```python
from build123d import *

# Parameters (mm, degrees)
SKETCH1_W   = 45.5
SKETCH1_H   = 37
BASIS_DEPTH = 4


with BuildPart() as part:
    # Sketch1 → Basis (new body)
    with BuildSketch(Plane.XY):
        with Locations((22.75, 18.5)):
            Rectangle(SKETCH1_W, SKETCH1_H)
        Polygon((14.5, 39.5), (12.5, 37), (16.5, 37), align=None)
        Polygon((31, 39.5), (29, 37), (33, 37), align=None)
        Polygon((16.5, 0), (12.5, 0), (14.5, -2.5), align=None)
        Polygon((33, 0), (29, 0), (31, -2.5), align=None)
    extrude(amount=BASIS_DEPTH)


solid = part.part
```
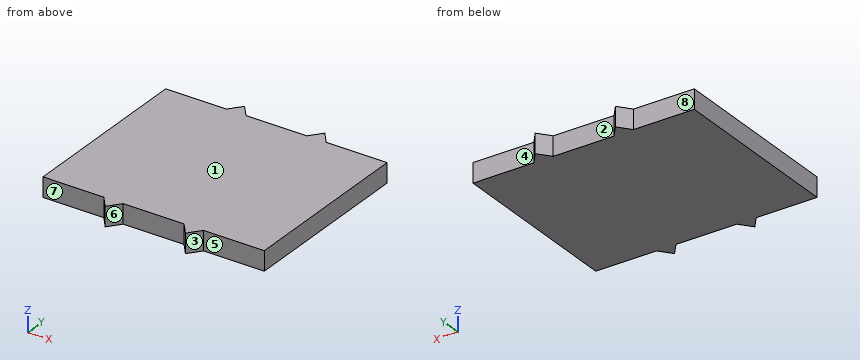
Read the model definition and answer for the solid it produces. Units are mm, in the model's axes. Face numbers are marked on the shaded views. A direction names the side the tool comes from. Give positions to 0.01 mm unless a question says otherwise; leave off trailing zeros. Write each loop counter-clockwise with the first axis right and the second up, starting at its lowest first coordinate (ties: lowest second). Pieces come first, ordered by that corner, then holes. Notation, with made-up numbers: (-38.5, -39) - (0.5, -39) arc R22 cw to (0.5, -31) - close; hole circle Ø9 at (74, 24.5). An arc over 180 degrees is marked (long way). Write item = value, one per line. Start each with the question number.
Item 1: Find section A-A (z = 3.4). Give the vertices of the cut face in (x, y), then the cut area to 3 significant figures.
Item 2: Find the intervals of material crossed by probe 1 along Y at (x, z) = (34.5, 3.2); probe 2 along Y at (x, z) = (15, 3.1) (3 decimals), in increasing order. Write a range as [from, to].
Item 3: The mould has two halves that part along X. Classify the marked faces 1, 2 and 3: +X half, -X half, draft (parallel to the pull), parting line (faces both ways), or undercut.
Item 4: Find section C-C (x = 13). Give the vertices of the cut face in (y, z) (3 decimals).
Item 5: This flat-tipped pin is pushed along its axis until it touches: P1, Ø1.2, axis at x = 39.5, z = 2, coming from the -Y side. Where does it stop, or does it pass through?
Item 6: Find section B-B (x = 36.5). Give the vertices of the cut face in (y, z).
Item 7: A tool of negligible diameter and unlimited length cuts with its end or side. For the marked faces 4, 5, 6, 7 and 8, from which of +Z, -Z, +X, -X, +Y, -Y can it reach the whole face along a straight path? Write none if from no direction.
Response:
q1.outline = (0, 0) - (12.5, 0) - (14.5, -2.5) - (16.5, 0) - (29, 0) - (31, -2.5) - (33, 0) - (45.5, 0) - (45.5, 37) - (33, 37) - (31, 39.5) - (29, 37) - (16.5, 37) - (14.5, 39.5) - (12.5, 37) - (0, 37) - close
q1.area = 1,700 mm²
q2.probe_1 = [0, 37]
q2.probe_2 = [-1.875, 38.875]
q3.face_1 = draft
q3.face_2 = undercut
q3.face_3 = +X half
q4.outline = (-0.625, 0) - (37.625, 0) - (37.625, 4) - (-0.625, 4) - close
q5.P1 = 0
q6.outline = (0, 0) - (37, 0) - (37, 4) - (0, 4) - close
q7.face_4 = +Z, -Z, +X, +Y
q7.face_5 = +Z, -Z, +X, -Y
q7.face_6 = +Z, -Z, -Y
q7.face_7 = +Z, -Z, -X, -Y
q7.face_8 = +Z, -Z, -X, +Y
